Source: three-view drawing plus pictorial views. Frame: mm from the lowest corner of the part. Coordinates: 2 decimals unless noted, no trailing zeros. Write each loop counter-clockwise with the first axis right and the second up, starting at its lowest first coordinate (ties: lowest second). Pieces come first, ordered by that corner, then holes. Notation, with made-up numbers: (-2.75, -3) -> (6.25, -3) arc R12 ccw to (6.25, 8) -> close; hole circle Ø3 at (20.5, 29). An arc over 180 degrees is marked (long way). One line per item, written item: value. Start each with the question number.
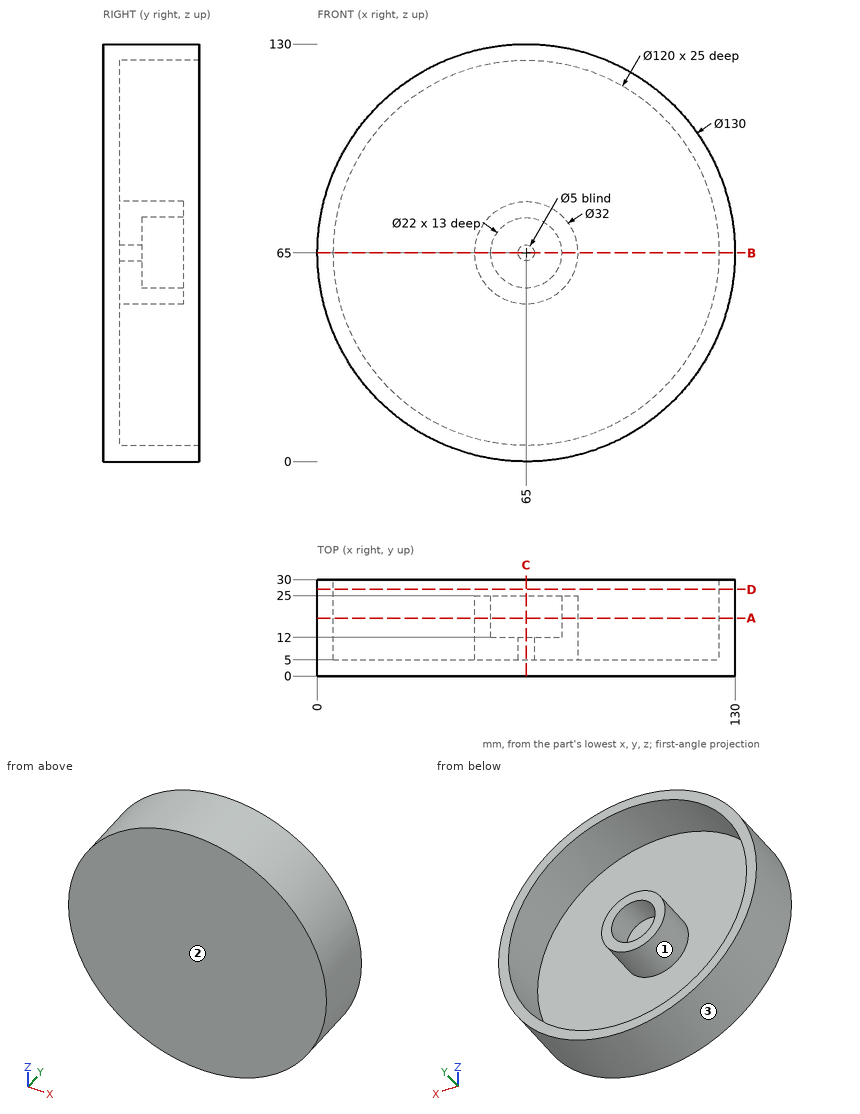
Q1. Cut plane B-B on z = 65. Output: boundary loops of the cut face in (x, y), and give its area (3 significant figures).
Q2. Draft query along Z for the marked faces 1, 2 and 3. Return one class per face: pulls with the +Z half, pulls with the -Z half, needs draft (parallel to the pull), parting line crosses it, or undercut.
Q3. Cut plane D-D on y = 27. Output: boundary loops of the cut face in (x, z).
Q4. Cut plane A-A on y = 18. Output: boundary loops of the cut face in (x, z).
Q5. First-contact query: P1, Ø10, axis at y = 13, z = 46, coming from the +X side; P2, Ø10, axis at x = 114, y = 23, coming from the -Z side; P3, Ø10, axis at x = 85, y = 24, coming from the +Z side; P4, Ø8, axis at x = 116, z = 114.5, coming from the -Y side. Flat tips, straight axial feed; report the tip coordinate or a pass-through.
Q6. Line query: L1, parallel to Z at x = 65, y = 16.5; L2, parallel to Z at x = 65, y = 9; L3, parallel to X at y = 13.75, z = 51. Output: solid intervals per line, ascending. Write a range as from..to.
Q7. Cut plane C-C on x = 65. Output: boundary loops of the cut face in (y, z), and give its area (3 significant figures).
Solution:
1. outline: (0, 0) -> (130, 0) -> (130, 30) -> (125, 30) -> (125, 5) -> (81, 5) -> (81, 25) -> (76, 25) -> (76, 12) -> (67.5, 12) -> (67.5, 5) -> (62.5, 5) -> (62.5, 12) -> (54, 12) -> (54, 25) -> (49, 25) -> (49, 5) -> (5, 5) -> (5, 30) -> (0, 30) -> close
1. area: 1,220 mm²
2. face 1: undercut
2. face 2: needs draft
2. face 3: parting line crosses it
3. outline: circle Ø130 at (65, 65); hole circle Ø120 at (65, 65)
4. outline: circle Ø130 at (65, 65); circle Ø32 at (65, 65); hole circle Ø120 at (65, 65); hole circle Ø22 at (65, 65)
5. P1: x = 128.47
5. P2: z = 17.16
5. P3: z = 128.25
5. P4: through
6. L1: 0..5, 49..54, 76..81, 125..130
6. L2: 0..5, 49..62.5, 67.5..81, 125..130
6. L3: 1.53..6.66, 57.25..72.75, 123.34..128.47
7. outline: (0, 0) -> (30, 0) -> (30, 5) -> (5, 5) -> (5, 49) -> (25, 49) -> (25, 54) -> (12, 54) -> (12, 62.5) -> (5, 62.5) -> (5, 67.5) -> (12, 67.5) -> (12, 76) -> (25, 76) -> (25, 81) -> (5, 81) -> (5, 125) -> (30, 125) -> (30, 130) -> (0, 130) -> close
7. area: 1,220 mm²
